Geometry check sheet. Reference: the model listing, model coordinates, mm. A direction names the side the tool comes from. Give positions to 0.01 mm unless a question says otherwise; leave off trailing zeros. Loops run counter-clockwise (first coordinate to the right, second up) from the corner with the lowest first, then second, coordinate; pieces in that order, holes last. Notation, with made-up numbers: (9, 88.25) - (17, 88.25) arc R19 cw to (17, 119.25) - close; hole circle Ø6 at (75, 81). An arc over 180 degrees is marked (long way). Write item = value, one per line. Start each with the question number.
from build123d import *

# Parameters (mm, degrees)
SKETCH1_R           = 2.15
BOSS_EXTRUDE1_DEPTH = 5
FILLET1_R           = 2


with BuildPart() as part:
    # Sketch1 → Boss-Extrude1 (new body)
    with BuildSketch(Plane(origin=(0, 0, 0), x_dir=(1, 0, 0), z_dir=(0, 1, 0))):
        with BuildLine():
            Line((60, -60), (-60, -60))
            Line((-60, -60), (-60, 60))
            Line((-60, 60), (-45, 60))
            ThreePointArc((-45, 60), (-30, 75), (-15, 60))
            Line((-15, 60), (15, 60))
            ThreePointArc((15, 60), (30, 45), (45, 60))
            Line((45, 60), (60, 60))
            Line((60, 60), (60, 45))
            ThreePointArc((60, 45), (75, 30), (60, 15))
            Line((60, 15), (60, -15))
            ThreePointArc((60, -15), (45, -30), (60, -45))
            Line((60, -45), (60, -60))
        make_face()
        with Locations(Location((-40, -40, 0), (0, 0, 270))):
            Circle(SKETCH1_R, mode=Mode.SUBTRACT)
        with Locations(Location((40, 40, 0), (0, 0, 270))):
            Circle(SKETCH1_R, mode=Mode.SUBTRACT)
        with Locations(Location((-40, 40, 0), (0, 0, 270))):
            Circle(SKETCH1_R, mode=Mode.SUBTRACT)
        with Locations(Location((0, 40, 0), (0, 0, 270))):
            Circle(SKETCH1_R, mode=Mode.SUBTRACT)
        with Locations(Location((-40, 0, 0), (0, 0, 270))):
            Circle(SKETCH1_R, mode=Mode.SUBTRACT)
        with Locations(Location((40, -40, 0), (0, 0, 270))):
            Circle(SKETCH1_R, mode=Mode.SUBTRACT)
        with Locations(Location((40, 0, 0), (0, 0, 270))):
            Circle(SKETCH1_R, mode=Mode.SUBTRACT)
        with Locations(Location((0, -40, 0), (0, 0, 270))):
            Circle(SKETCH1_R, mode=Mode.SUBTRACT)
    extrude(amount=BOSS_EXTRUDE1_DEPTH)

    # Fillet1
    fillet1_edges = [part.edges().sort_by_distance(p)[0] for p in [
        (-45, 2.5, -60),
        (-15, 2.5, -60),
        (15, 2.5, -60),
        (45, 2.5, -60),
        (60, 2.5, -45),
        (60, 2.5, -15),
        (60, 2.5, 15),
        (60, 2.5, 45),
    ]]
    fillet(fillet1_edges, radius=FILLET1_R)


solid = part.part
1) Cross-section at C-C on y = 2.65. Give the number of separate pieces and of enclosed holes in the cut face, and give its area (3 significant figures).
2) Cross-section at D-D on x = 0. Enter the section's corners in (y, z), and give its area (3 significant figures).
3) Release check for a two-part mould opening along Z. For faces 1 (the face through (60, 2, 0)), 2 (the face through (-54, 2, -60)), 3 (the face through (-37.87, 2.46, -0.28)) record: pulls with the +Z half, pulls with the -Z half, needs draft (parallel to the pull), parting line crosses it, or undercut.
4) Tool access check on faces 4 (the face through (0.65, 2.46, -37.95)), 5 (the face through (0, 2, -60)), 6 (the face through (60, 2, 53)). Record the directions out of +Z, -Z, +X, -X, +Y, -Y that give a thin tool (end or side, any length) a straight path to the whole face; none if there is none.
5) Cross-section at A-A on x = 51. Enter the section's corners in (y, z), and give its area (3 significant figures).
6) Cross-section at B-B on z = 0. Enter the section's corners in (x, y), and give its area (3 significant figures).
7) Gauge pin test, flat ends, axial feed: P1, Ø1.5, axis at x = -54.5, y = 3, coming from the -Z side; P2, Ø3, axis at x = 35.5, y = 3, coming from the -Z side. Record the tip position at first contact, or that the pin passes through.
8) Material ranges on line 1 along X through (y, z) = (2.25, 0); line 2 along X through (y, z) = (3.05, -1); line 3 along X through (y, z) = (2.2, -40), recorded low to high.
Checked values:
q1.separate_pieces = 1
q1.enclosed_holes = 8
q1.area = 14,300 mm²
q2.outline = (0, -60) - (5, -60) - (5, -42.15) - (0, -42.15) - close; (0, -37.85) - (5, -37.85) - (5, 37.85) - (0, 37.85) - close; (0, 42.15) - (5, 42.15) - (5, 60) - (0, 60) - close
q2.area = 557 mm²
q3.face_1 = needs draft
q3.face_2 = pulls with the -Z half
q3.face_3 = undercut
q4.face_4 = +Y, -Y
q4.face_5 = -Z, +X, +Y, -Y
q4.face_6 = +Z, +X, +Y, -Y
q5.outline = (0, -60) - (5, -60) - (5, 18) - (0, 18) - close; (0, 42) - (5, 42) - (5, 60) - (0, 60) - close
q5.area = 480 mm²
q6.outline = (-60, 0) - (-42.15, 0) - (-42.15, 5) - (-60, 5) - close; (-37.85, 0) - (37.85, 0) - (37.85, 5) - (-37.85, 5) - close; (42.15, 0) - (60, 0) - (60, 5) - (42.15, 5) - close
q6.area = 557 mm²
q7.P1 = -60
q7.P2 = -46.73
q8.line_1 = -60 to -42.15, -37.85 to 37.85, 42.15 to 60
q8.line_2 = -60 to -41.9, -38.1 to 38.1, 41.9 to 60
q8.line_3 = -60 to -42.15, -37.85 to -2.15, 2.15 to 37.85, 42.15 to 71.18
